Design review of the part built by this model. Coordinates are the model's own, in mm. A direction names the side the tool comes from. Coordinates: 2 decimals unless noted, no trailing zeros. Loops run counter-clockwise (first coordinate to the right, second up) from the corner with the lowest first, then second, coordinate; pieces in that order, holes last. Notation, with made-up numbers: (83.5, 75.25) -> (139.5, 75.25) arc R9 ccw to (139.5, 81.25) -> close; hole circle Ø3 at (32.25, -2.75). An arc over 180 degrees is marked (long way). Answer as a JSON object with one key per item and string values.
```python
from build123d import *

# Parameters (mm, degrees)
F1_DEPTH = 304.8


with BuildPart() as f1:
    # F0 (on Front) → F1 (new body)
    with BuildSketch(Plane.XZ):
        with BuildLine():
            Line((0, 53.001386), (0, 0))
            Line((0, 0), (177.8, 0))
            Line((177.8, 0), (177.8, 53.001386))
            ThreePointArc((177.8, 53.001386), (173.582811, 50.892435), (171.413937, 46.705748))
            Line((171.413937, 46.705748), (165.679132, 11.926927))
            ThreePointArc((165.679132, 11.926927), (163.004781, 7.204374), (157.910044, 5.334))
            Line((157.910044, 5.334), (19.889956, 5.334))
            ThreePointArc((19.889956, 5.334), (14.795219, 7.204374), (12.120868, 11.926927))
            Line((12.120868, 11.926927), (6.386063, 46.705748))
            ThreePointArc((6.386063, 46.705748), (4.217189, 50.892435), (0, 53.001386))
        make_face()
    extrude(amount=F1_DEPTH)


solid = f1.part
```
1) Add section A-A, the plane z = 38. Give the boundary of the cut face in (x, y).
Completed:
{"outline": "(0, -304.8) -> (7.82, -304.8) -> (7.82, 0) -> (0, 0) -> close; (169.98, -304.8) -> (177.8, -304.8) -> (177.8, 0) -> (169.98, 0) -> close"}
2) Add section D-D, the plane x = 106. Give the boundary of the cut face in (y, z), and give its area (3 significant figures).
Completed:
{"outline": "(-304.8, 0) -> (0, 0) -> (0, 5.33) -> (-304.8, 5.33) -> close", "area": "1,630 mm²"}
3) Clearance check with a flat-ended pin moving along its axis: pin 1 Ø1.5 at (x, y) = (138, -199) entering from +Z. State where the tip first meets the part, or that it passes through.
Completed:
{"pin 1": "z = 5.33"}
4) The part is to be moulded in two halves that separate along X. For faces 1 (the flat face through (0, -150, 27)), 2 (the flat face through (88, -150, 0)), 3 (the flat face through (177.8, -150, 26)), 4 (the cylindrical face through (14.855, -150.266, 7.154)), say which applies: pulls with the +X half, pulls with the -X half, needs draft (parallel to the pull), parting line crosses it, or undercut.
Completed:
{"face 1": "pulls with the -X half", "face 2": "needs draft", "face 3": "pulls with the +X half", "face 4": "undercut"}
5) Add section C-C, the plane z = 21.5. Give the boundary of the cut face in (x, y).
Completed:
{"outline": "(0, -304.8) -> (10.54, -304.8) -> (10.54, 0) -> (0, 0) -> close; (167.26, -304.8) -> (177.8, -304.8) -> (177.8, 0) -> (167.26, 0) -> close"}
6) Wall thickness on probe 1 along Z at (x, y) = (31, -91); probe 2 along X at (y, z) = (-218.5, 31.5); probe 3 along X at (y, z) = (-21, 20): over which ranges is each line inside the solid? List them lowest first.
Completed:
{"probe 1": "0 to 5.33", "probe 2": "0 to 8.89, 168.91 to 177.8", "probe 3": "0 to 10.79, 167.01 to 177.8"}
7) Add section B-B, the plane y = -220.5. Give the boundary of the cut face in (x, z).
Completed:
{"outline": "(0, 0) -> (177.8, 0) -> (177.8, 53) arc R7.62 ccw to (171.41, 46.71) -> (165.68, 11.93) arc R7.87 cw to (157.91, 5.33) -> (19.89, 5.33) arc R7.87 cw to (12.12, 11.93) -> (6.39, 46.71) arc R7.62 ccw to (0, 53) -> close"}
8) For faces 5 (the cylindrical face through (4.26, -150.27, 50.85)), 6 (the flat face through (88, -304.8, 5)), list the 3-axis set-ups (+Z, -Z, +X, -X, +Y, -Y) from which the entire face can be reached by the end or side of a thin tool; tool diameter is ignored.
Completed:
{"face 5": "+Z, +Y, -Y", "face 6": "+Z, -Z, +X, -X, -Y"}
